Source: CAD feature listing. Evaluate the final solid. Frame: model axes, mm. A direction names the side the tool comes from. Coordinates: 2 decimals unless noted, no trailing zeros. Write each loop counter-clockwise with the first axis right and the second up, starting at its lowest first coordinate (ties: lowest second). Pieces come first, ordered by that corner, then holes. Notation, with made-up numbers: (3, 44.25) - (16, 44.25) arc R17 cw to (16, 67.25) - close; hole circle Ø8 at (-15.75, 28.5). An arc over 180 degrees is marked (long way). One line per item, written item: value.
from build123d import *

# Parameters (mm, degrees)
IZIM2_R                     = 5
Y_KSEKLIK_EKSTR_ZYON2_DEPTH = 10
IZIM3_W                     = 140
IZIM3_H                     = 10
Y_KSEKLIK_EKSTR_ZYON3_DEPTH = 40
IZIM4_R                     = 5
Y_KSEKLIK_EKSTR_ZYON4_DEPTH = 10
IZIM5_R                     = 5
KES_EKSTR_ZYON1_DEPTH       = 10


with BuildPart() as part:
    # Çizim2 → Yükseklik-Ekstrüzyon2 (new body)
    with BuildSketch(Plane.XY):
        with BuildLine():
            Line((-49.137152365, 3.922510102), (-49.137152365, -6.077489898))
            Line((-49.137152365, -6.077489898), (90.862847635, -6.077489898))
            Line((90.862847635, -6.077489898), (90.862847635, 3.922510102))
            ThreePointArc((90.862847635, 3.922510102), (62.578576387, 15.638238855), (50.862847635, 43.922510102))
            Line((50.862847635, 43.922510102), (-9.137152365, 43.922510102))
            ThreePointArc((-9.137152365, 43.922510102), (-20.852881118, 15.638238855), (-49.137152365, 3.922510102))
        make_face()
        with Locations((5.862847635, 33.922510102)):
            Circle(IZIM2_R, mode=Mode.SUBTRACT)
        with Locations((35.862847635, 33.922510102)):
            Circle(IZIM2_R, mode=Mode.SUBTRACT)
    extrude(amount=Y_KSEKLIK_EKSTR_ZYON2_DEPTH)

    # Çizim3 → Yükseklik-Ekstrüzyon3 (add)
    with BuildSketch(Plane.XY.offset(10)):
        with Locations((20.862847635, -1.077489898)):
            Rectangle(IZIM3_W, IZIM3_H)
    extrude(amount=Y_KSEKLIK_EKSTR_ZYON3_DEPTH)

    # Çizim4 → Yükseklik-Ekstrüzyon4 (add)
    with BuildSketch(Plane.XY.offset(50)):
        with BuildLine():
            Line((-49.137152365, 3.922510102), (-49.137152365, -6.077489898))
            Line((-49.137152365, -6.077489898), (90.862847635, -6.077489898))
            Line((90.862847635, -6.077489898), (90.862847635, 3.922510102))
            ThreePointArc((90.862847635, 3.922510102), (62.578576387, 15.638238855), (50.862847635, 43.922510102))
            Line((50.862847635, 43.922510102), (-9.137152365, 43.922510102))
            ThreePointArc((-9.137152365, 43.922510102), (-20.852881118, 15.638238855), (-49.137152365, 3.922510102))
        make_face()
        with Locations((5.862847635, 33.922510102)):
            Circle(IZIM4_R, mode=Mode.SUBTRACT)
        with Locations((35.862847635, 33.922510102)):
            Circle(IZIM4_R, mode=Mode.SUBTRACT)
    extrude(amount=Y_KSEKLIK_EKSTR_ZYON4_DEPTH)

    # Çizim5 → Kes-Ekstrüzyon1 (cut)
    with BuildSketch(Plane(origin=(0, 3.922510102, 0), x_dir=(1, 0, 0), z_dir=(0, 1, 0))):
        with Locations(Location((20.862847635, -30, 0), (0, 0, 270))):
            Circle(IZIM5_R)
    extrude(amount=-KES_EKSTR_ZYON1_DEPTH, mode=Mode.SUBTRACT)


solid = part.part
1) Contact query for flat-ended pins moving along their axis: P1, Ø6, axis at x = 73.5, z = 53.5, coming from the +Y side; P2, Ø12, axis at y = 38, z = 52, coming from the +X side; P3, Ø12, axis at x = 39.5, z = 37.5, coming from the +Y side. Output: stop coordinate, or through.
Values found:
P1: y = 9.49
P2: x = 52.68
P3: y = 3.92
2) Section query A-A on z = 30. Output: boundary loops of the cut face in (x, y).
Values found:
outline: (-49.14, -6.08) - (15.86, -6.08) - (15.86, 3.92) - (-49.14, 3.92) - close; (25.86, -6.08) - (90.86, -6.08) - (90.86, 3.92) - (25.86, 3.92) - close
3) Draft query along Z for faces 1 (the flat face through (20, 20, 10)), 2 (the cylindrical face through (21, -1, 25)), 3 (the cylindrical face through (30.868, 34.142, 54.93)), 4 (the flat face through (20, 14, 60)). Return one class per face: released by +Z, released by -Z, zero draft, split by the parting line, or undercut.
Values found:
face 1: undercut
face 2: undercut
face 3: zero draft
face 4: released by +Z
4) Reachability of faces 5 (the cylindrical face through (30.868, 34.142, 4.93)), 6 (the flat face through (20, 20, 50)) from +Z, -Z, +X, -X, +Y, -Y: full face, straight path, thin tool, end or side. Return the list, or none.
Values found:
face 5: +Z, -Z
face 6: +X, -X, +Y
5) Material intervals for line 1 (Z direction, x = -16.5, y = 20.5); line 2 (X direction, y = -2.5, z = 30); line 3 (Y direction, x = -15.5, z = 21), sorted ascending.
Values found:
line 1: 0 to 10, 50 to 60
line 2: -49.14 to 15.86, 25.86 to 90.86
line 3: -6.08 to 3.92
6) Section query D-D on z = 6. Output: boundary loops of the cut face in (x, y).
Values found:
outline: (-49.14, -6.08) - (90.86, -6.08) - (90.86, 3.92) arc R40 cw to (50.86, 43.92) - (-9.14, 43.92) arc R40 cw to (-49.14, 3.92) - close; hole circle Ø10 at (5.86, 33.92); hole circle Ø10 at (35.86, 33.92)
7) Section query C-C on y = 21. Output: boundary loops of the cut face in (x, z), then the cut area to 3 significant figures.
Values found:
outline: (-16.36, 0) - (58.08, 0) - (58.08, 10) - (-16.36, 10) - close; (-16.36, 50) - (58.08, 50) - (58.08, 60) - (-16.36, 60) - close
area: 1,490 mm2
8) Section query B-B on x = 33. Output: boundary loops of the cut face in (y, z), then the cut area to 3 significant figures.
Values found:
outline: (-6.08, 0) - (29.82, 0) - (29.82, 10) - (3.92, 10) - (3.92, 50) - (29.82, 50) - (29.82, 60) - (-6.08, 60) - close; (38.02, 0) - (43.92, 0) - (43.92, 10) - (38.02, 10) - close; (38.02, 50) - (43.92, 50) - (43.92, 60) - (38.02, 60) - close
area: 1,240 mm2
